Geometry check sheet. Reference: the model listing, model coordinates, mm. Face numbers are marked on the shaded views. Give positions to 0.01 mm unless a question says otherwise; leave off trailing zeros. Loops run counter-clockwise (first coordinate to the right, second up) from the corner with the lowest first, then second, coordinate; pieces in that order, holes last. Notation, with made-up numbers: (-1, -19) - (54, -19) arc R30 cw to (54, 7) - close; hole circle Ø3 at (52, 85). An arc over 180 degrees is marked (long way). Use a Markdown table: item, result. Add a question column.
1. Cross-section at C-C on z = -16. Enter the section's corners in (x, y).
2. Material ranges on L1, parallel to Y at x = 0, z = -84; L2, parallel to X at y = 0.5, z = -68; L3, parallel to Z at x = -2, y = -16, recorded low to high.
3. Draft check along Y on the marked faces 1, 2 and 3. Enter one of: pulls with the +Y half, pulls with the -Y half, needs draft (parallel to the pull), parting line crosses it, or undercut.
4. Cross-section at A-A on y = 0. Enter the section's corners in (x, z), and give its area (3 significant figures).
5. Depth check by flat-ended pin: P1, Ø6, axis at x = 5, y = 17.5, coming from the +Z side; P2, Ø1, axis at x = -1.5, z = -12, coming from the +Y side; P3, Ø6, axis at x = 5.5, z = -32, coming from the +Y side; P4, Ø6, axis at x = 10, z = -70, coming from the -Y side. Enter the tip coordinate at first touch or a pass-through.
6. Cross-section at D-D on x = 10. Enter the section's corners in (y, z), and give its area (3 significant figures).
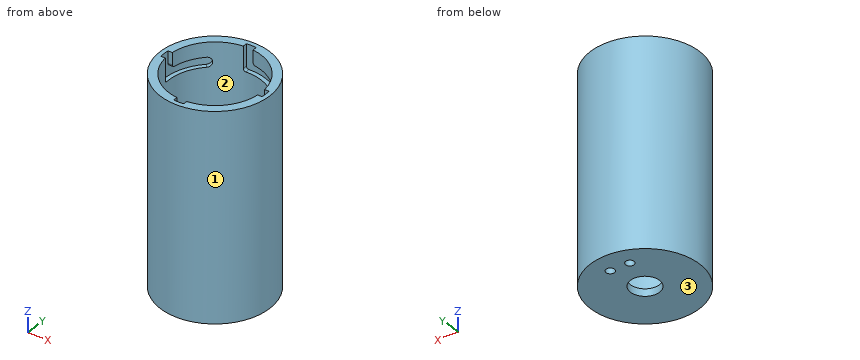
from build123d import *
from OCP.BRepFilletAPI import BRepFilletAPI_MakeFillet

# Parameters (mm, degrees)
SKETCH1_R                  = 22.5
SKETCH1_R_2                = 19
BOSS_EXTRUDE2_DEPTH        = 85
BOSS_EXTRUDE5_START        = -3
SKETCH3_R                  = 19
SKETCH3_R_2                = 6
BOSS_EXTRUDE5_DEPTH        = 3
CUT_EXTRUDE1_DEPTH         = 10
CUT_REVOLVE2_ANGLE         = 52.00000000000012
FILLET2_R                  = 2
FILLET2_R_2                = 1
CIRPATTERN1_COUNT          = 4
FILLET2_OF_CIRPATTERN1_R   = 2
FILLET2_OF_CIRPATTERN1_R_2 = 1
SKETCH17_R                 = 1.7499999999999998
CUT_EXTRUDE2_DEPTH         = 10


with BuildPart() as part:
    # Sketch1 → Boss-Extrude2 (new body)
    with BuildSketch(Plane.XY):
        Circle(SKETCH1_R)
        Circle(SKETCH1_R_2, mode=Mode.SUBTRACT)
    extrude(amount=-BOSS_EXTRUDE2_DEPTH)

    # Sketch3 → Boss-Extrude5 (add)
    with BuildSketch(Plane(origin=(0, 0, -85), x_dir=(-1, 0, 0), z_dir=(0, 0, -1)).offset(BOSS_EXTRUDE5_START)):
        with Locations(Location((0, 0, 0), (0, 0, 180))):
            Circle(SKETCH3_R)
        Circle(SKETCH3_R_2, mode=Mode.SUBTRACT)
    extrude(amount=BOSS_EXTRUDE5_DEPTH)

    # Sketch4 → Cut-Extrude1 (cut)
    with BuildSketch(Plane.XY):
        with BuildLine():
            ThreePointArc((1.999999999999999, 20.653389552322885), (1.27e-15, 20.75), (-2.000000000000001, 20.65338955232288))
            Line((-2, 20.65338955232288), (-2, 18.894443627691185))
            ThreePointArc((-2.000000000000001, 18.894443627691185), (1.16e-15, 19), (1.999999999999999, 18.894443627691185))
            Line((2, 18.894443627691185), (2, 20.65338955232288))
        make_face()
    cut_extrude1 = extrude(amount=-CUT_EXTRUDE1_DEPTH, mode=Mode.SUBTRACT)

    # Sketch8 → Cut-Revolve2 (revolve, cut)
    with BuildSketch(Plane(origin=(0, 0, 0), x_dir=(0, 0, -1), z_dir=(1, 0, 0))):
        Polygon((6.000000000000001, 20.75), (10, 20.75), (10, 18.9), (6.000000000000002, 18.9), align=None)
    cut_revolve2 = revolve(axis=Axis((0, 0, 0), (0, 0, -1)), revolution_arc=CUT_REVOLVE2_ANGLE, mode=Mode.SUBTRACT)

    # Fillet2
    fillet2_edges_1 = [part.edges().sort_by_distance(p)[0] for p in [
        (15.661713727933623, 12.236271822097425, -6.000000000000001),
        (15.661713727933623, 12.236271822097425, -10),
    ]]
    fillet2_edges_2 = [part.edges().sort_by_distance(p)[0] for p in [
        (-2, 19.773916590007033, -10),
        (2, 19.773916590007033, -6.000000000000002),
    ]]
    fillet2 = BRepFilletAPI_MakeFillet(part.part.solid().wrapped)
    for e in fillet2_edges_1:
        fillet2.Add(FILLET2_R - 0.0001, e.wrapped)
    for e in fillet2_edges_2:
        fillet2.Add(FILLET2_R_2 - 0.0001, e.wrapped)
    add(Compound.cast(fillet2.Shape()), mode=Mode.REPLACE)  # a hair under: the kernel refuses the full size

    # CirPattern1: Cut-Extrude1, Cut-Revolve2 ×4 about axis
    cirpattern1_axis = Axis((0, 0, 0), (0, 0, 1))
    add([cut_extrude1.rotate(cirpattern1_axis, i * 360 / CIRPATTERN1_COUNT) for i in range(1, CIRPATTERN1_COUNT)], mode=Mode.SUBTRACT)
    add([cut_revolve2.rotate(cirpattern1_axis, i * 360 / CIRPATTERN1_COUNT) for i in range(1, CIRPATTERN1_COUNT)], mode=Mode.SUBTRACT)

    # Fillet2 of CirPattern1
    fillet2_of_cirpattern1_edges_1 = [part.edges().sort_by_distance(p)[0] for p in [
        (-12.236271822097423, 15.661713727933625, -6.000000000000001),
        (-12.236271822097423, 15.661713727933627, -10),
        (-15.661713727933625, -12.236271822097423, -6.000000000000001),
        (-15.661713727933627, -12.236271822097423, -10),
        (12.236271822097422, -15.661713727933629, -6.000000000000001),
        (12.236271822097422, -15.661713727933627, -10),
    ]]
    fillet2_of_cirpattern1_edges_2 = [part.edges().sort_by_distance(p)[0] for p in [
        (-19.773916590007033, -1.9999999999999978, -10),
        (-19.773916590007033, 2.000000000000002, -6.000000000000002),
        (1.9999999999999976, -19.773916590007033, -10),
        (-2.000000000000002, -19.773916590007033, -6.000000000000002),
        (19.773916590007033, 1.9999999999999956, -10),
        (19.773916590007033, -2.000000000000004, -6.000000000000002),
    ]]
    fillet2_of_cirpattern1 = BRepFilletAPI_MakeFillet(part.part.solid().wrapped)
    for e in fillet2_of_cirpattern1_edges_1:
        fillet2_of_cirpattern1.Add(FILLET2_OF_CIRPATTERN1_R - 0.0001, e.wrapped)
    for e in fillet2_of_cirpattern1_edges_2:
        fillet2_of_cirpattern1.Add(FILLET2_OF_CIRPATTERN1_R_2 - 0.0001, e.wrapped)
    add(Compound.cast(fillet2_of_cirpattern1.Shape()), mode=Mode.REPLACE)  # a hair under: the kernel refuses the full size

    # Sketch17 → Cut-Extrude2 (cut)
    with BuildSketch(Plane(origin=(0, 0, -85), x_dir=(-1, 0, 0), z_dir=(0, 0, -1))):
        with Locations((-4, 14.16)):
            Circle(SKETCH17_R)
        with Locations((4, 14.16)):
            Circle(SKETCH17_R)
    extrude(amount=-CUT_EXTRUDE2_DEPTH, mode=Mode.SUBTRACT)


solid = part.part
Values found:
| question | item | result |
|---|---|---|
| 1 | outline | circle Ø45 at (0, 0); hole circle Ø38 at (0, 0) |
| 2 | L1 | y = -22.5 to -6, 6 to 22.5 |
| 2 | L2 | x = -22.49 to -18.99, 18.99 to 22.49 |
| 2 | L3 | z = -85 to -82 |
| 3 | face 1 | parting line crosses it |
| 3 | face 2 | undercut |
| 3 | face 3 | needs draft |
| 4 | outline | (-22.5, -85) - (-6, -85) - (-6, -82) - (-19, -82) - (-19, -10) - (-20.75, -10) - (-20.75, 0) - (-22.5, 0) - close; (6, -85) - (22.5, -85) - (22.5, 0) - (20.75, 0) - (20.75, -10) - (19, -10) - (19, -82) - (6, -82) - close |
| 4 | area | 638 mm2 |
| 5 | P1 | stops at z = 0 |
| 5 | P2 | stops at y = 22.48 |
| 5 | P3 | stops at y = 22.36 |
| 5 | P4 | stops at y = -21.38 |
| 6 | outline | (-20.16, -85) - (20.16, -85) - (20.16, 0) - (16.16, 0) - (16.16, -6) - (18.18, -6) - (18.18, -10) - (16.16, -10) - (16.16, -82) - (-16.16, -82) - (-16.16, 0) - (-20.16, 0) - close |
| 6 | area | 769 mm2 |
